Source: CAD feature listing. Evaluate the final solid. Frame: model axes, mm. A direction names the side the tool comes from. Give positions to 0.01 mm unless a question says otherwise; leave off trailing zeros. Write each loop counter-clockwise with the first axis right and the second up, starting at its lowest first coordinate (ties: lowest second). Pieces come first, ordered by that corner, then holes. Notation, with made-up numbers: M 3,-13 L 14,-13 A24 cw 14,7 Z; hole C -13.5,71 d7. An arc over 180 degrees is marked long. Use CSV: the item, a comma, the result in double quotes. Start each with the question number.
from build123d import *

# Parameters (mm, degrees)
SKETCH1_W               = 250
SKETCH1_H               = 350
BOSS_EXTRUDE1_DEPTH     = 10
SKETCH2_W               = 248
SKETCH2_H               = 348
CUT_EXTRUDE1_DEPTH      = 9
CUT_EXTRUDE2_DEPTH      = 431.232495286
CUT_EXTRUDE2_DEPTH_BACK = 431.232495286
SKETCH3_R               = 2.5
SKETCH4_W               = 99
SKETCH4_H               = 61
CUT_EXTRUDE3_DEPTH      = 10
CUT_EXTRUDE4_REACH      = 432.232
SKETCH5_R               = 6.2


with BuildPart() as part:
    # Sketch1 → Boss-Extrude1 (new body)
    with BuildSketch(Plane.XY):
        with Locations((125, -175)):
            Rectangle(SKETCH1_W, SKETCH1_H)
    extrude(amount=BOSS_EXTRUDE1_DEPTH)

    # Sketch2 → Cut-Extrude1 (cut)
    with BuildSketch(Plane(origin=(0, 0, 0), x_dir=(-1, 0, 0), z_dir=(0, 0, -1))):
        with Locations((-125, -175)):
            Rectangle(SKETCH2_W, SKETCH2_H)
    extrude(amount=-CUT_EXTRUDE1_DEPTH, mode=Mode.SUBTRACT)

    # Sketch3 → Cut-Extrude2 (cut, two sides: drawn at the far end of the back side and taken through both)
    with BuildSketch(Plane(origin=(0, 0, 0), x_dir=(1, 0, 0), z_dir=(0, 1, 0)).offset(-CUT_EXTRUDE2_DEPTH_BACK)):
        with Locations(Location((7.5, -5, 0), (0, 0, 270))):
            Circle(SKETCH3_R)
    extrude(amount=CUT_EXTRUDE2_DEPTH + CUT_EXTRUDE2_DEPTH_BACK, mode=Mode.SUBTRACT)

    # Sketch4 → Cut-Extrude3 (cut)
    with BuildSketch(Plane.XY.offset(10)):
        with Locations((125, -90.5)):
            Rectangle(SKETCH4_W, SKETCH4_H)
    extrude(amount=-CUT_EXTRUDE3_DEPTH, mode=Mode.SUBTRACT)

    # Sketch5 → Cut-Extrude4 (cut, up to next)
    with BuildSketch(Plane.XY.offset(10), mode=Mode.PRIVATE) as cut_extrude4_sk1:
        with Locations((108.8, -156)):
            Circle(SKETCH5_R)
    cut_extrude4_tool1 = extrude(cut_extrude4_sk1.sketch, amount=-CUT_EXTRUDE4_REACH, mode=Mode.PRIVATE) & part.part
    # Sketch5 → Cut-Extrude4 (cut, up to next)
    with BuildSketch(Plane.XY.offset(10), mode=Mode.PRIVATE) as cut_extrude4_sk2:
        with Locations((141.2, -156)):
            Circle(SKETCH5_R)
    cut_extrude4_tool2 = extrude(cut_extrude4_sk2.sketch, amount=-CUT_EXTRUDE4_REACH, mode=Mode.PRIVATE) & part.part
    # Sketch5 → Cut-Extrude4 (cut, up to next)
    with BuildSketch(Plane.XY.offset(10), mode=Mode.PRIVATE) as cut_extrude4_sk3:
        with Locations((76.4, -156)):
            Circle(SKETCH5_R)
    cut_extrude4_tool3 = extrude(cut_extrude4_sk3.sketch, amount=-CUT_EXTRUDE4_REACH, mode=Mode.PRIVATE) & part.part
    # Sketch5 → Cut-Extrude4 (cut, up to next)
    with BuildSketch(Plane.XY.offset(10), mode=Mode.PRIVATE) as cut_extrude4_sk4:
        with Locations(Location((173.6, -156, 0), (0, 0, 180))):
            Circle(SKETCH5_R)
    cut_extrude4_tool4 = extrude(cut_extrude4_sk4.sketch, amount=-CUT_EXTRUDE4_REACH, mode=Mode.PRIVATE) & part.part
    add(cut_extrude4_tool1.solids().sort_by_distance((108.8, -156, 10))[0], mode=Mode.SUBTRACT)
    add(cut_extrude4_tool2.solids().sort_by_distance((141.2, -156, 10))[0], mode=Mode.SUBTRACT)
    add(cut_extrude4_tool3.solids().sort_by_distance((76.4, -156, 10))[0], mode=Mode.SUBTRACT)
    add(cut_extrude4_tool4.solids().sort_by_distance((173.6, -156, 10))[0], mode=Mode.SUBTRACT)


solid = part.part
1. Line query: probe 1 along Y at (x, z) = (141.2, 9.85); probe 2 along Y at (x, z) = (87, 3); probe 3 along X at (y, z) = (-0.35, 5). Output: solid intervals per line, ascending.
2. Section A-A on y = -156. Return loops of the section in (x, z), then the cut area to 3 significant figures.
3. Access query for faces 5 (the cylindrical face through (75.056, -162.053, 9.507)), 6 (the flat face through (127, -349, 4)). Directions: +Z, -Z, +X, -X, +Y, -Y. A direction counts if a zero-diameter tool reaches every point of the face in a straight line with its end or side. Return the directions, or none.
4. Section B-B on x = 92.5. Return loops of the section in (y, z), then the cut area to 3 significant figures.
5. Section C-C on z = 5. Return loops of the section in (x, y), then the cut area to 3 significant figures.
6. First-contact query: pin 1 (16 mm diameter, centred on x = 173.6, y = -156, fed in from -Z). Flat tip, straight axial feed; report the tip coordinate or a pass-through.
7. Section D-D on y = -68. Return loops of the section in (x, z), then the cut area to 3 significant figures.
8. Pull-direction query (X, two-part tool) for faces 1 (the flat face through (0, -177, 5)), 2 (the flat face through (250, -177, 5)), 3 (the flat face through (123, -173, 10)), 4 (the cylindrical face through (107.456, -162.053, 9.507)); classes: released by +X, released by -X, zero draft, split by the parting line, or undercut.
Resolved:
1,probe 1,"y = -350 to -162.2, -149.8 to -121, -60 to 0"
1,probe 2,"y = -350 to -349, -1 to 0"
1,probe 3,"x = 0 to 5, 10 to 250"
2,outline,"M 0,0 L 1,0 L 1,9 L 70.2,9 L 70.2,10 L 0,10 Z; M 82.6,9 L 102.6,9 L 102.6,10 L 82.6,10 Z; M 115,9 L 135,9 L 135,10 L 115,10 Z; M 147.4,9 L 167.4,9 L 167.4,10 L 147.4,10 Z; M 179.8,9 L 249,9 L 249,0 L 250,0 L 250,10 L 179.8,10 Z"
2,area,"218 mm2"
3,face 5,"+Z, -Z"
3,face 6,"-Z"
4,outline,"M -350,0 L -349,0 L -349,9 L -121,9 L -121,10 L -350,10 Z; M -60,9 L -1,9 L -1,0 L 0,0 L 0,10 L -60,10 Z"
4,area,"307 mm2"
5,outline,"M 0,-350 L 5,-350 L 5,-349 L 1,-349 L 1,-1 L 5,-1 L 5,0 L 0,0 Z; M 10,-350 L 250,-350 L 250,0 L 10,0 L 10,-1 L 249,-1 L 249,-349 L 10,-349 Z"
5,area,"1,190 mm2"
6,pin 1,"stops at z = 9"
7,outline,"M 0,0 L 1,0 L 1,9 L 75.5,9 L 75.5,10 L 0,10 Z; M 174.5,9 L 249,9 L 249,0 L 250,0 L 250,10 L 174.5,10 Z"
7,area,"169 mm2"
8,face 1,"released by -X"
8,face 2,"released by +X"
8,face 3,"zero draft"
8,face 4,"undercut"
